from build123d import *

# Parameters (mm, degrees)
F0_W        = 85
F0_H        = 10
F0_R        = 1.5
F1_DEPTH    = 4
F2_T1_DEPTH = 34.4948974279
F3_R        = 2


# Not quite as in the source:
# - a fillet or chamfer that OpenCascade refuses, or shapes differently, is made with other operations: its cross-section is extruded or revolved along the edge and cut away or added


with BuildPart() as f1:
    # F0 (on Top) → F1 (new body)
    with BuildSketch(Plane.XY):
        with Locations((5.8581340313, 5)):
            Rectangle(F0_W, F0_H)
        with BuildLine():
            ThreePointArc((-24.6418659687, 6.5), (-23.5812057969, 6.0606601718), (-23.1418659687, 5))
            ThreePointArc((-23.1418659687, 5), (-23.5812057969, 3.9393398282), (-24.6418659687, 3.5))
            ThreePointArc((-24.6418659687, 3.5), (-26.1418659687, 5), (-24.6418659687, 6.5))
        make_face(mode=Mode.SUBTRACT)
        with Locations((-4.6418659687, 5)):
            Circle(F0_R, mode=Mode.SUBTRACT)
        with Locations((15.3581340313, 5)):
            Circle(F0_R, mode=Mode.SUBTRACT)
        with Locations((35.3581340313, 5)):
            Circle(F0_R, mode=Mode.SUBTRACT)
    extrude(amount=F1_DEPTH)

    # F2: fillet of radius 5 on 2 edges, made by hand

    # F2_s2 → F2_t1 (cut)
    with BuildSketch(Plane.XZ.offset(-22.2474487139)):
        with BuildLine():
            ThreePointArc((-31.7428864831, 4), (-34.9051641433, 2.8729833462), (-36.6418659687, 0))
            Line((-36.6418659687, 0), (-36.6418659687, 4))
            Line((-36.6418659687, 4), (-31.7428864831, 4))
        make_face()
        with BuildLine():
            ThreePointArc((43.4591545457, 4), (46.6214322059, 2.8729833462), (48.3581340313, 0))
            Line((48.3581340313, 0), (48.3581340313, 4))
            Line((48.3581340313, 4), (43.4591545457, 4))
        make_face()
    extrude(amount=F2_T1_DEPTH, mode=Mode.SUBTRACT)

    # F3
    f3_edges = [f1.edges().sort_by_distance(p)[0] for p in [
        (5.858134, 10, 4),
        (5.858134, 0, 4),
        (-34.905164, 10, 2.872983),
        (46.621432, 10, 2.872983),
        (-34.905164, 0, 2.872983),
        (46.621432, 0, 2.872983),
    ]]
    fillet(f3_edges, radius=F3_R)


solid = f1.part
Verification items for the finished model (mm, model axes). Give positions to 0.01 mm unless a question says otherwise; leave off trailing zeros. Loops run counter-clockwise (first coordinate to the right, second up) from the corner with the lowest first, then second, coordinate; pieces in that order, holes last.
1. Release check for a two-part mould opening along X. For faces 1 (the cylindrical face through (-3.21, 5.45, 1.97)), 2 (the cylindrical face through (33.86, 5.07, 1.97)), 3 (the cylindrical face through (46.584, 5.042, 2.903)), 4 (the cylindrical face through (6.38, 0.57, 3.4)) record: +X half, -X half, draft (parallel to the pull), parting line (faces both ways), or undercut.
Derived:
face 1: undercut
face 2: undercut
face 3: +X half
face 4: draft
2. Material ranges on probe 1 along X at (y, z) = (5.5, 1.95); probe 2 along Y at (x, z) = (13, 2.2); probe 3 along Y at (x, z) = (-24, 2.7), recorded low to high.
Derived:
probe 1: x = -35.78 to -26.06, -23.23 to -6.06, -3.23 to 13.94, 16.77 to 33.94, 36.77 to 47.5
probe 2: y = 0.01 to 9.99
probe 3: y = 0.13 to 3.64, 6.36 to 9.87
3. Cross-section at C-C on z = 0.85. Count the separate pieces of the cut face and the enclosed holes in it, and give its area (3 significant figures).
Derived:
separate pieces: 1
enclosed holes: 4
area: 813 mm2
4. Cross-section at B-B on x = -14. Record the cut outline in (y, z).
Derived:
outline: (0, 0) - (10, 0) - (10, 2) arc R2 ccw to (8, 4) - (2, 4) arc R2 ccw to (0, 2) - close
5. Cross-section at A-A on x = -5. Record the cut outline in (y, z).
Derived:
outline: (0, 0) - (3.54, 0) - (3.54, 4) - (2, 4) arc R2 ccw to (0, 2) - close; (6.46, 0) - (10, 0) - (10, 2) arc R2 ccw to (8, 4) - (6.46, 4) - close
6. Go/stop test with flat-tipped pins: P1, Ø4, axis at x = 15.36, y = 5, coming from the -Z side; P2, Ø2, axis at y = 8, z = 3, coming from the +X side. Record where each tip stops, or that it passes through.
Derived:
P1: stops at z = 0
P2: stops at x = 47.46
